```python
from build123d import *

# Parameters (mm, degrees)
BOSS_EXTRUDE2_DEPTH = 5
BOSS_EXTRUDE3_START = -5
BOSS_EXTRUDE3_DEPTH = 5
SKETCH5_W           = 1.5
SKETCH5_H           = 7.215071269
BOSS_EXTRUDE4_DEPTH = 5


with BuildPart() as part:
    # Sketch1 → Boss-Extrude2 (new body)
    with BuildSketch(Plane(origin=(0, 0, 0), x_dir=(1, 0, 0), z_dir=(0, 1, 0))):
        with BuildLine():
            Line((-35, 10.092006525), (-35, 34.126916803))
            ThreePointArc((-35, 34.126916803), (-42.067915891, 17.063458401), (-35, 0))
            ThreePointArc((-35, 0), (-17.5, -2.732905818), (0, 0))
            ThreePointArc((0, 0), (7.067915891, 17.063458401), (0, 34.126916803))
            Line((0, 34.126916803), (0, 11.021533442))
            ThreePointArc((0, 11.021533442), (-17.776697358, 20.975411278), (-35, 10.092006525))
        make_face()
    extrude(amount=BOSS_EXTRUDE2_DEPTH)

    # Sketch4 → Boss-Extrude3 (add)
    with BuildSketch(Plane(origin=(0, 5, 0), x_dir=(1, 0, 0), z_dir=(0, 1, 0)).offset(BOSS_EXTRUDE3_START)):
        with BuildLine():
            Line((0, 0), (0, -7.215071269))
            Line((0, -7.215071269), (-35, -7.215071269))
            Line((-35, -7.215071269), (-35, 0))
            ThreePointArc((-35, 0), (-42.067915891, 17.063458401), (-35, 34.126916803))
            Line((-35, 34.126916803), (-35, 10.092006525))
            ThreePointArc((-35, 10.092006525), (-17.776697358, 20.975411278), (0, 11.021533442))
            Line((0, 11.021533442), (0, 34.126916803))
            ThreePointArc((0, 34.126916803), (7.067915891, 17.063458401), (0, 0))
        make_face()
    extrude(amount=BOSS_EXTRUDE3_DEPTH)

    # Sketch5 → Boss-Extrude4 (add)
    with BuildSketch(Plane(origin=(0, 5, 0), x_dir=(1, 0, 0), z_dir=(0, 1, 0))):
        with Locations((-35.75, -3.607535635)):
            Rectangle(SKETCH5_W, SKETCH5_H)
        with Locations((0.75, -3.607535635)):
            Rectangle(SKETCH5_W, SKETCH5_H)
    extrude(amount=-BOSS_EXTRUDE4_DEPTH)


solid = part.part
```
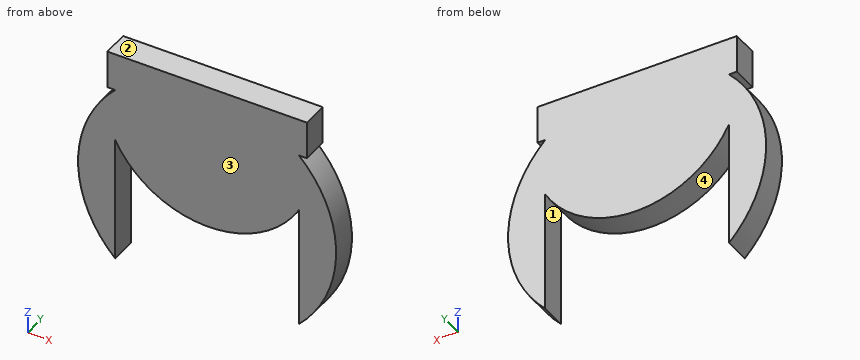
Here's how the part is built. I have some questions about the finished solid (model axes, mm). Face numbers are marked on the shaded views. A direction names the side the tool comes from. Give positions to 0.01 mm unless a question says otherwise; leave off trailing zeros. Loops run counter-clockwise (first coordinate to the right, second up) from the corner with the lowest first, then second, coordinate; pieces in that order, holes last. Notation, with made-up numbers: M -29.5,-38.5 L 17.5,-38.5 A18 ccw 17.5,-34.5 Z; hole C 14,6 d5. An arc over 180 degrees is marked long. Return JSON: item names as keys, results as strings.
Item 1: Thinking about a two-plate mould opening in X: for the marked faces 3 and 4, which applies, released by +X, released by -X, zero draft, split by the parting line, or undercut?
A:
{"face 3": "zero draft", "face 4": "undercut"}
Item 2: Imagine slicing it at C-C on x = -25.5. List the corners of the cut face in (y, z) for me.
A:
{"outline": "M 0,-19.19 L 5,-19.19 L 5,7.22 L 0,7.22 Z"}
Item 3: Imagine slicing it at D-D on z = -31. List the corners of the cut face in (x, y) for me, then the cut area to 3 significant figures.
A:
{"outline": "M -37.64,0 L -35,0 L -35,5 L -37.64,5 Z; M 0,0 L 2.64,0 L 2.64,5 L 0,5 Z", "area": "26.4 mm^2"}
Item 4: Imagine slicing it at B-B on z = -25. List the corners of the cut face in (x, y) for me.
A:
{"outline": "M -40.73,0 L -35,0 L -35,5 L -40.73,5 Z; M 0,0 L 5.73,0 L 5.73,5 L 0,5 Z"}
Item 5: On a 3-axis mill with a long thin cutter (end or side, diameter ignored), from which of +Z, -Z, +X, -X, +Y, -Y can I reach the whole of each face in a straight line? I mean the marked faces 1 and 2. Say none if no direction works.
A:
{"face 1": "-Z, +Y, -Y", "face 2": "+Z, +X, -X, +Y, -Y"}
Item 6: I'm going to push flat-ended pins straight in: pin 1 Ø1 at (y, z) = (1, -24.5) entering from +X; pin 2 Ø1 at (y, z) = (4, -27) entering from -X; pin 3 Ø2.5 at (y, z) = (2.5, -24) entering from -X; pin 4 Ø12 at (x, z) = (-18, -22.5) entering from -Y. Where does each tip first touch, or does it pass through?
A:
{"pin 1": "stops at x = 6.05", "pin 2": "stops at x = -40.15", "pin 3": "stops at x = -41.39", "pin 4": "stops at y = 0"}
Item 7: Imagine slicing it at A-A on y = 1.5. List the corners of the cut face in (x, z) for me.
A:
{"outline": "M -36.5,0 L -35,0 A24.13 ccw -35,-34.13 L -35,-10.09 A19.91 ccw 0,-11.02 L 0,-34.13 A24.13 ccw 0,0 L 1.5,0 L 1.5,7.22 L -36.5,7.22 Z"}
Item 8: Please list where these lines run through material, in increasing order: line 1 (X direction, y = 2.85, z = -17.5); line 2 (X direction, y = 2.6, z = -16); line 3 (X direction, y = 2.25, z = 1).
A:
{"line 1": "x = -42.06 to -35, -28.5 to -6, 0 to 7.06", "line 2": "x = -42.04 to -35, -30.42 to -4.07, 0 to 7.04", "line 3": "x = -36.5 to 1.5"}
